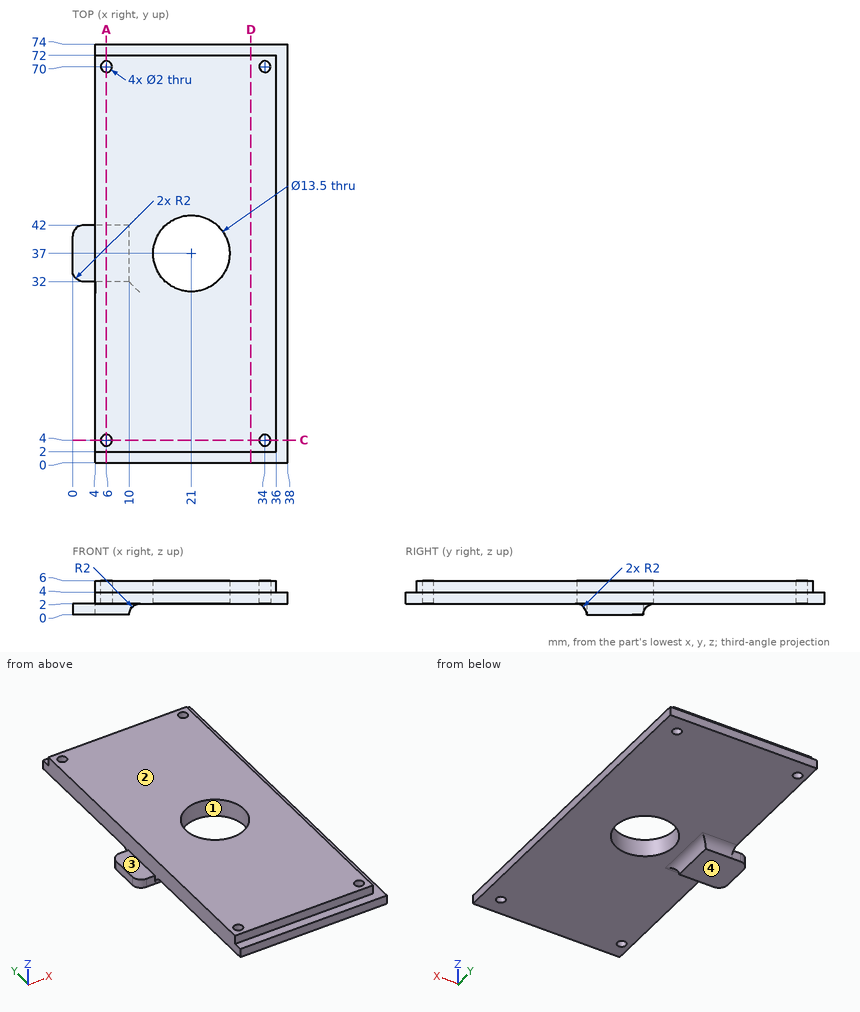
Here's the drawing with two shaded views (mm, measured from the low corner). I have some questions. A direction names the side the tool comes from. Give positions to 0.01 mm unless a question says otherwise; leave off trailing zeros. Write each loop counter-clockwise with the first axis right and the second up, starting at its lowest first coordinate (ties: lowest second). Pieces come first, ordered by that corner, then holes. Notation, with made-up numbers: (18, -28) -> (67, -28) arc R32 ccw to (67, 5) -> close; hole circle Ø7 at (73.5, 87.5). An arc over 180 degrees is marked (long way). Use one line per item in the form item = value. Start each with the question number.
1. On a 3-axis mill with a long thin cutter (end or side, diameter ignored), from which of +Z, -Z, +X, -X, +Y, -Y can I reach the whole of each face in a straight line? I mean the marked faces 3 and 4. Say none if no direction works.
2. If I drill on L1, parallel to Y at x = 6, z = 3.3; L2, parallel to X at y = 70, z = 4.7; L3, parallel to Y at x = 34, z = 4.95, over which ranges is the centre line in solid material (lowest first)?
3. Imagine slicing it at A-A on x = 6. State how many separate pieces and enclosed holes the cut face has, plus the area to 3 significant figures.
4. Imagine slicing it at C-C on y = 4. List the corners of the cut face in (x, z) for me.
5. Imagine slicing it at D-D on x = 31.5. List the corners of the cut face in (y, z) for me, plus the area to 3 significant figures.
6. Thinking about a two-plate mould opening in X: for the marked faces 1 and 2, which applies, +X half, -X half, draft (parallel to the pull), parting line (faces both ways), or undercut?
7. Will these pins go through, and if not, where does the flat tip stop? pin 1 Ø1.8 at (x, y) = (34, 4) entering from +Z; pin 2 Ø1 at (x, z) = (7, 1) entering from -Y; pin 3 Ø3 at (x, y) = (6, 70) entering from -Z; pin 4 Ø3 at (x, y) = (1.5, 39) entering from +Z.
Entries:
q1.face_3 = +Z, -X, +Y, -Y
q1.face_4 = -Z, +X, -X, +Y, -Y
q2.L1 = 0 to 3, 5 to 69, 71 to 74
q2.L2 = 4 to 5, 7 to 33, 35 to 36
q2.L3 = 2 to 3, 5 to 69, 71 to 72
q3.separate_pieces = 3
q3.enclosed_holes = 0
q3.area = 294 mm²
q4.outline = (4, 2) -> (5, 2) -> (5, 6) -> (4, 6) -> close; (7, 2) -> (33, 2) -> (33, 6) -> (7, 6) -> close; (35, 2) -> (38, 2) -> (38, 4) -> (36, 4) -> (36, 6) -> (35, 6) -> close
q5.outline = (0, 2) -> (74, 2) -> (74, 4) -> (72, 4) -> (72, 6) -> (2, 6) -> (2, 4) -> (0, 4) -> close
q5.area = 288 mm²
q6.face_1 = undercut
q6.face_2 = draft
q7.pin_1 = through
q7.pin_2 = 31.32
q7.pin_3 = 2
q7.pin_4 = 2
